The listing builds one solid part. Answer for the finished solid, in the listing's coordinates (mm). Round coordinates to 2 decimals unless told otherwise and drop trailing zeros. Loops run counter-clockwise (first coordinate to the right, second up) from the corner with the lowest first, then second, coordinate; pieces in that order, holes last. Notation, with made-up numbers: (23, 18.5) - (43, 18.5) arc R19 cw to (43, 50.5) - close; hole circle Ø6 at (80.25, 84.5). An arc over 180 degrees is marked (long way). Write item = value, one per line. Start each with the question number.
1) Straight lines are drawn through the part: line 1 along X through (y, z) = (120, -1); line 2 along X through (y, z) = (115, -0.15); line 3 along Y through (x, z) = (-22.5, -1.95). For each, find the intervals that lie inside material, in ascending order.
2) Section A-A, the plane z = -2.4 is taken. Determine the outline of the cut face in (x, y) (1 decimal).
3) Section B-B, the plane x = -34.5 is taken. Determine the outline of the cut face in (y, z) (3 decimals), and give its area (3 significant figures).
4) Section C-C, the plane y = 110.25 is taken. Determine the outline of the cut face in (x, z) (3 decimals), and give its area (3 significant figures).
5) Given pin 1 Ø1 at (y, z) = (107.5, -2) entering from -X; pin 2 Ø1 at (y, z) = (112.5, -2) entering from -X, each flat-ended and moving along its own axis, determine where each tip first touches the part or whether it passes through.
from build123d import *

# Parameters (mm, degrees)
SKETCH1_R           = 0.635
BOSS_EXTRUDE1_DEPTH = 3.175


with BuildPart() as part:
    # Sketch1 → Boss-Extrude1 (new body)
    with BuildSketch(Plane.XY):
        Polygon((-1.5875, 113.111399164), (-1.5875, 128.504233601), (-170.312713847, 120.085477895), (-171.411810426, 103.527545161), align=None)
        with Locations((-156.924194119, 107.841267283)):
            Circle(SKETCH1_R, mode=Mode.SUBTRACT)
        with Locations((-8.346623216, 122.968890993)):
            Circle(SKETCH1_R, mode=Mode.SUBTRACT)
    extrude(amount=-BOSS_EXTRUDE1_DEPTH)


solid = part.part
Geometry check:
q1.line_1 = -170.32 to -1.59
q1.line_2 = -170.65 to -1.59
q1.line_3 = 111.93 to 127.46
q2.outline = (-171.4, 103.5) - (-1.6, 113.1) - (-1.6, 128.5) - (-170.3, 120.1) - close; hole circle Ø1.3 at (-156.9, 107.8); hole circle Ø1.3 at (-8.3, 123)
q3.outline = (111.254, -3.175) - (126.862, -3.175) - (126.862, 0) - (111.254, 0) - close
q3.area = 49.6 mm2
q4.outline = (-170.966, -3.175) - (-52.291, -3.175) - (-52.291, 0) - (-170.966, 0) - close
q4.area = 377 mm2
q5.pin_1 = -171.18
q5.pin_2 = -170.85
